Geometry check sheet. Reference: drawing and pictorial views, mm from the part's lowest x, y, z. A direction names the side the tool comes from. Round coordinates to 2 decimals unless told otherwise and drop trailing zeros. Loops run counter-clockwise (first coordinate to the right, second up) from the corner with the lowest first, then second, coordinate; pieces in that order, holes last. Notation, with made-up numbers: (-16.75, 14) - (20.25, 14) arc R27 ccw to (20.25, 52) - close; hole circle Ø3 at (38.25, -32). An arc over 180 degrees is marked (long way). Return JSON: item names as keys, results as strings.
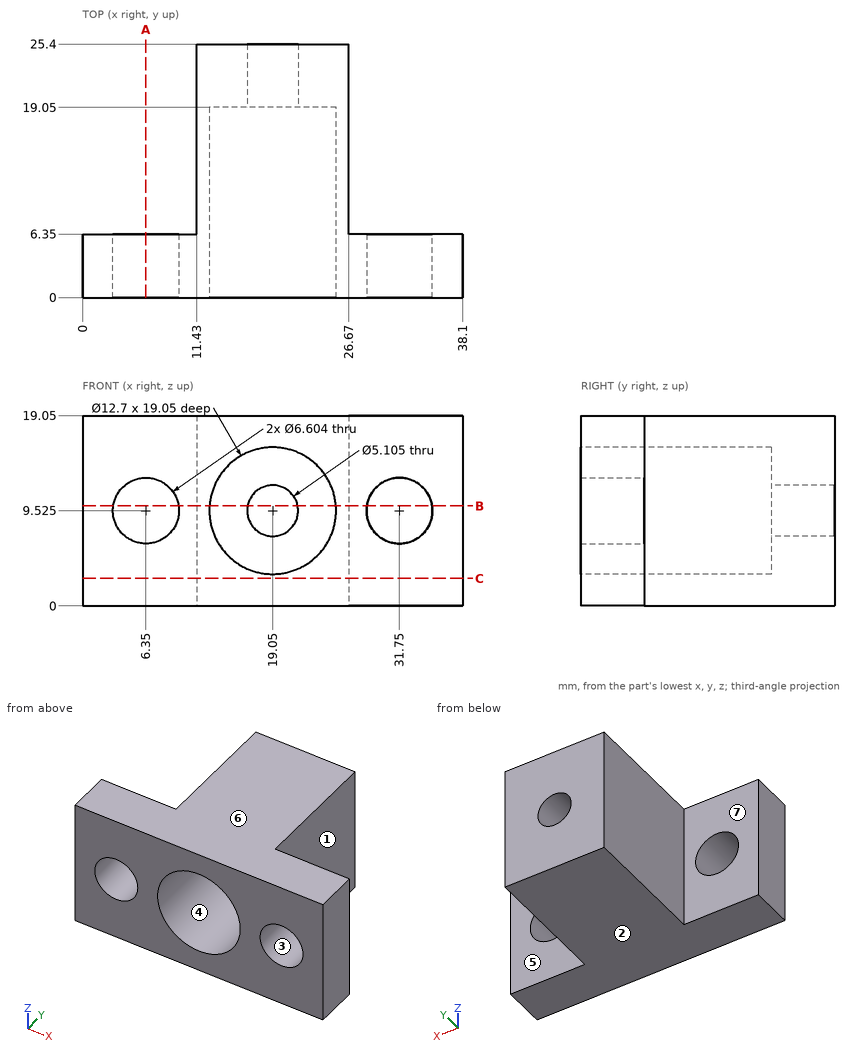
Q1. Sectioned sample at C-C (z = 2.75). Enter the section's corners in (x, y), plus the area to 3 significant figures.
Answer key:
{"outline": "(0, 0) - (38.1, 0) - (38.1, 6.35) - (26.67, 6.35) - (26.67, 25.4) - (11.43, 25.4) - (11.43, 6.35) - (0, 6.35) - close", "area": "532 mm²"}
Q2. Scan lines: probe 1 along Z at (x, y) = (19.05, 21.75); probe 2 along X at (y, z) = (6.25, 6.75); probe 3 along Y at (x, z) = (3, 7.25). Record each from-to range of solid material in increasing order. Write a range as [from, to].
Answer key:
{"probe 1": "z = [0, 6.97], [12.08, 19.05]", "probe 2": "x = [0, 4.56], [8.14, 13.34], [24.76, 29.96], [33.54, 38.1]", "probe 3": "y = [0, 6.35]"}
Q3. Sectioned sample at B-B (z = 10). Enter the section's corners in (x, y), plus the area to 3 significant figures.
Answer key:
{"outline": "(0, 0) - (3.08, 0) - (3.08, 6.35) - (0, 6.35) - close; (9.62, 0) - (12.72, 0) - (12.72, 19.05) - (16.54, 19.05) - (16.54, 25.4) - (11.43, 25.4) - (11.43, 6.35) - (9.62, 6.35) - close; (21.56, 19.05) - (25.38, 19.05) - (25.38, 0) - (28.48, 0) - (28.48, 6.35) - (26.67, 6.35) - (26.67, 25.4) - (21.56, 25.4) - close; (35.02, 0) - (38.1, 0) - (38.1, 6.35) - (35.02, 6.35) - close", "area": "176 mm²"}
Q4. Draft check along Z on the marked faces 1, 2, 3 and 4. Enter one of: released by +Z, released by -Z, zero draft, split by the parting line, or undercut.
Answer key:
{"face 1": "zero draft", "face 2": "released by -Z", "face 3": "undercut", "face 4": "undercut"}
Q5. Depth check by flat-ended pin: P1, Ø3.5, axis at x = 6, z = 6, coming from the +Y side; P2, Ø4, axis at x = 16.5, z = 7, coming from the -Y side; P3, Ø4.5, axis at x = 19.05, z = 9.525, coming from the +Y side; P4, Ø2, axis at y = 18, z = 2.5, coming from the -X side. Enter the tip coordinate at first touch or a pass-through.
Answer key:
{"P1": "stops at y = 6.35", "P2": "stops at y = 19.05", "P3": "passes through", "P4": "stops at x = 11.43"}
Q6. Tool access check on the marked faces 5, 6 and 7. Record the directions out of +Z, -Z, +X, -X, +Y, -Y that give a thin tool (end or side, any length) a straight path to the whole face; none if there is none.
Answer key:
{"face 5": "+Z, -Z, +X, +Y", "face 6": "+Z, +X, -X, +Y, -Y", "face 7": "+Z, -Z, -X, +Y"}
Q7. Sectioned sample at A-A (x = 6.35). Enter the section's corners in (y, z).
Answer key:
{"outline": "(0, 0) - (6.35, 0) - (6.35, 6.22) - (0, 6.22) - close; (0, 12.83) - (6.35, 12.83) - (6.35, 19.05) - (0, 19.05) - close"}
